Here's how the part is built. I have some questions about the finished solid (model axes, mm). Face numbers are marked on the shaded views. A direction names the side the tool comes from. Coordinates: 2 decimals unless noted, no trailing zeros. Order: outer loops, then holes, each group sorted by start corner. A loop starts at its lowest first (then second) coordinate and runs counter-clockwise, first axis right, second up. Notation, with made-up numbers: (3.5, 84.25) - (16.5, 84.25) arc R17 ccw to (16.5, 110.25) - close; hole circle Ø4 at (75, 68.5). An arc over 180 degrees is marked (long way). Answer as CSV lines item,"result". Start each with the question number.
Item 1: I need wall thicknesses on line 1 (Z direction, x = -0.5, y = 3.75); line 2 (Y direction, x = -0.5, z = -4.5); line 3 (Y direction, x = -0.5, z = -7.75). Which ranges of each line are inside material? Lowest first, please.
Item 2: We'd pull the mould along Y, two halves only. Please class the marked faces 6, 7 and 8: pulls with the +Y half, pulls with the -Y half, needs draft (parallel to the pull), parting line crosses it, or undercut.
Item 3: On a 3-axis mill with a long thin cutter (end or side, diameter ignored), from which of +Z, -Z, +X, -X, +Y, -Y can I reach the whole of each face in a straight line? I mean the marked faces 1, 2, 3, 4 and 5. Say none if no direction works.
Item 4: Imagine slicing it at C-C on z = -8.5. List the corners of the cut face in (x, y) for me.
Item 5: Imagine slicing it at D-D on x = 1. List the corners of the cut face in (y, z) for me, and give its area (3 significant figures).
Item 6: Imagine slicing it at A-A on z = -5.5. List the corners of the cut face in (x, y) for me, and give its area (3 significant figures).
Item 7: I'm going to push flat-ended pins straight in: pin 1 (2 mm diameter, centred on x = -1, z = -5, fed in from +Y); pin 2 (3.5 mm diameter, centred on y = 7, z = -9.5, fed in from +X); pin 3 (1 mm diameter, centred on x = 0.5, y = 0.5, fed in from +Z); pin 4 (0.7 mm diameter, centred on y = 1, z = -6, fed in from +X). Where does each tip first touch, or does it pass through?
Item 8: Imagine slicing it at B-B on y = 5.75. List the corners of the cut face in (x, z) for me, and give its area (3 significant figures).
from build123d import *

# Parameters (mm, degrees)
SKICA1_W                = 6.5
SKICA1_H                = 6.5
P_IDAT_VYSUNUT_M1_DEPTH = 13
SKICA2_W                = 4
SKICA2_H                = 4
P_IDAT_VYSUNUT_M2_DEPTH = 3.5
SKICA3_W                = 1.3
SKICA3_H                = 0.7
SKICA5_W                = 1.3
SKICA5_H                = 0.8
SKICA7_W                = 1.3
SKICA7_H                = 0.8


with BuildPart() as part:
    # Skica1 → Přidat vysunutím1 (new body)
    with BuildSketch(Plane(origin=(0, 0, 0), x_dir=(1, 0, 0), z_dir=(0, 1, 0))):
        Rectangle(SKICA1_W, SKICA1_H)
    extrude(amount=P_IDAT_VYSUNUT_M1_DEPTH)

    # Skica2 → Přidat vysunutím2 (add)
    with BuildSketch(Plane.XY.offset(3.25)):
        with Locations((0, 5)):
            Rectangle(SKICA2_W, SKICA2_H)
    extrude(amount=P_IDAT_VYSUNUT_M2_DEPTH)

    # Táhnout po křivce1: sweep along a path in Skica4
    with BuildLine(Plane(origin=(0, 0, 0), x_dir=(0, 0, -1), z_dir=(1, 0, 0))) as t_hnout_po_k_ivce1_path:
        Line((3.25, 11.05), (14.45, 11.05))
        ThreePointArc((14.45, 11.05), (15.015685425, 10.815685425), (15.25, 10.25))
        Line((15.25, 10.25), (15.25, 0))
    # Skica3 → Táhnout po křivce1 (sweep)
    with BuildSketch(Plane(origin=(0, 0, -3.25), x_dir=(-1, 0, 0), z_dir=(0, 0, -1))):
        with Locations((0, 11.05)):
            Rectangle(SKICA3_W, SKICA3_H)
    sweep(path=t_hnout_po_k_ivce1_path.line)

    # Táhnout po křivce2: sweep along a path in Skica6
    with BuildLine(Plane(origin=(0, 0, 0), x_dir=(0, 0, -1), z_dir=(1, 0, 0))) as t_hnout_po_k_ivce2_path:
        Line((3.25, 6.8), (10.45, 6.8))
        ThreePointArc((10.45, 6.8), (11.015685425, 6.565685425), (11.25, 6))
        Line((11.25, 6), (11.25, 0))
    # Skica5 → Táhnout po křivce2 (sweep)
    with BuildSketch(Plane(origin=(0, 0, -3.25), x_dir=(-1, 0, 0), z_dir=(0, 0, -1))):
        with Locations((0, 6.8)):
            Rectangle(SKICA5_W, SKICA5_H)
    sweep(path=t_hnout_po_k_ivce2_path.line)

    # Táhnout po křivce3: sweep along a path in Skica8
    with BuildLine(Plane(origin=(0, 0, 0), x_dir=(0, 0, -1), z_dir=(1, 0, 0))) as t_hnout_po_k_ivce3_path:
        Line((3.25, 2), (6.45, 2))
        ThreePointArc((6.45, 2), (7.015685425, 1.765685425), (7.25, 1.2))
        Line((7.25, 1.2), (7.25, 0))
    # Skica7 → Táhnout po křivce3 (sweep)
    with BuildSketch(Plane(origin=(0, 0, -3.25), x_dir=(-1, 0, 0), z_dir=(0, 0, -1))):
        with Locations((0, 2)):
            Rectangle(SKICA7_W, SKICA7_H)
    sweep(path=t_hnout_po_k_ivce3_path.line)


solid = part.part
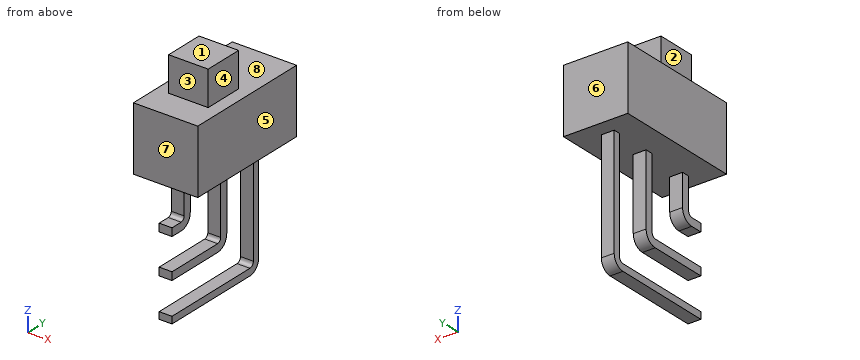
Responses:
1,line 1,"z = -15.6 to -14.9, -11.65 to -10.85, -3.25 to 6.75"
1,line 2,"y = 1.6 to 2.4, 6.4 to 7.2, 10.7 to 11.4"
1,line 3,"y = 6.4 to 7.2, 10.7 to 11.4"
2,face 6,"pulls with the +Y half"
2,face 7,"pulls with the -Y half"
2,face 8,"needs draft"
3,face 1,"+Z, +X, -X, +Y, -Y"
3,face 2,"+Z, -X, +Y, -Y"
3,face 3,"+Z, +X, -X, -Y"
3,face 4,"+Z, +X, +Y, -Y"
3,face 5,"+Z, -Z, +X, +Y, -Y"
4,outline,"(-0.65, 6.4) - (0.65, 6.4) - (0.65, 7.2) - (-0.65, 7.2) - close; (-0.65, 10.7) - (0.65, 10.7) - (0.65, 11.4) - (-0.65, 11.4) - close"
5,outline,"(0, -3.25) - (13, -3.25) - (13, 3.25) - (7, 3.25) - (7, 6.75) - (3, 6.75) - (3, 3.25) - (0, 3.25) - close"
5,area,"98.5 mm^2"
6,outline,"(-0.65, 1.6) - (0.65, 1.6) - (0.65, 2.4) - (-0.65, 2.4) - close; (-0.65, 6.4) - (0.65, 6.4) - (0.65, 7.2) - (-0.65, 7.2) - close; (-0.65, 10.7) - (0.65, 10.7) - (0.65, 11.4) - (-0.65, 11.4) - close"
6,area,"2.99 mm^2"
7,pin 1,"stops at y = 11.4"
7,pin 2,"stops at x = 0.65"
7,pin 3,"stops at z = 3.25"
7,pin 4,"passes through"
8,outline,"(-3.25, -3.25) - (3.25, -3.25) - (3.25, 3.25) - (2, 3.25) - (2, 6.75) - (-2, 6.75) - (-2, 3.25) - (-3.25, 3.25) - close; (-0.65, -15.6) - (0.65, -15.6) - (0.65, -14.9) - (-0.65, -14.9) - close; (-0.65, -11.65) - (0.65, -11.65) - (0.65, -10.85) - (-0.65, -10.85) - close"
8,area,"58.2 mm^2"
